from build123d import *

# Parameters (mm, degrees)
F1_DEPTH = 66.675
F2_R     = 1.5875
F2_R_2   = 11.1125
F3_DEPTH = 25.401
F4_R     = 2.8575
F5_DEPTH = 3.556
F6_R     = 3.302
F7_DEPTH = 50.801


with BuildPart() as f1:
    # F0 (on Front) → F1 (new body)
    with BuildSketch(Plane.XZ):
        Polygon((0, 50.8), (0, 0), (25.4, 0), (25.4, 6.35), (6.35, 6.35), (6.35, 50.8), align=None)
    extrude(amount=F1_DEPTH)

    # F2 (on face) → F3 (cut, through all)
    with BuildSketch(Plane(origin=(0, 0, 0), x_dir=(0, -1, 0), z_dir=(-1, 0, 0))):
        with Locations((19.05, 25.4)):
            Circle(F2_R)
        with Locations((33.3375, 39.6875)):
            Circle(F2_R)
        with Locations((33.3375, 25.4)):
            Circle(F2_R_2)
        with Locations((47.625, 25.4)):
            Circle(F2_R)
        with Locations((33.3375, 11.1125)):
            Circle(F2_R)
    extrude(amount=-F3_DEPTH, mode=Mode.SUBTRACT)

    # F4 (on face) → F5 (cut)
    with BuildSketch(Plane(origin=(0, 0, 0), x_dir=(0, -1, 0), z_dir=(-1, 0, 0))):
        with Locations((33.3375, 39.6875)):
            Circle(F4_R)
        with Locations((47.625, 25.4)):
            Circle(F4_R)
        with Locations((33.3375, 11.1125)):
            Circle(F4_R)
        with Locations((19.05, 25.4)):
            Circle(F4_R)
    extrude(amount=-F5_DEPTH, mode=Mode.SUBTRACT)

    # F6 (on face) → F7 (cut, through all)
    with BuildSketch(Plane(origin=(0, 0, 0), x_dir=(1, 0, 0), z_dir=(0, 0, -1))):
        with Locations((12.7, 9.652)):
            Circle(F6_R)
        with Locations((12.7, 57.023)):
            Circle(F6_R)
    extrude(amount=-F7_DEPTH, mode=Mode.SUBTRACT)


solid = f1.part
Verification items for the finished model (mm, model axes). A direction names the side the tool comes from. Give positions to 0.01 mm unless a question says otherwise; leave off trailing zeros. Loops run counter-clockwise (first coordinate to the right, second up) from the corner with the lowest first, then second, coordinate; pieces in that order, holes last.
1. Cross-section at A-A on z = 25.4. Count the separate pieces of the cut face and the enclosed holes in it, and give its area (3 significant figures).
Derived:
separate pieces: 4
enclosed holes: 0
area: 224 mm2
2. Cross-section at C-C on y = -19.05. Record the cut outline in (x, z).
Derived:
outline: (0, 0) - (25.4, 0) - (25.4, 6.35) - (6.35, 6.35) - (6.35, 23.81) - (3.56, 23.81) - (3.56, 22.54) - (0, 22.54) - close; (0, 28.26) - (3.56, 28.26) - (3.56, 26.99) - (6.35, 26.99) - (6.35, 50.8) - (0, 50.8) - close
3. Go/stop test with flat-tipped pins: P1, Ø3.5, axis at y = -47.625, z = 25.4, coming from the -X side; P2, Ø8.5, axis at x = 12.7, y = -57.023, coming from the +Z side; P3, Ø1.9, axis at y = -47.625, z = 25.4, coming from the -X side; P4, Ø5, axis at y = -33.34, z = 11.11, coming from the +X side. Record where each tip stops, or that it passes through.
Derived:
P1: stops at x = 3.56
P2: stops at z = 6.35
P3: passes through
P4: stops at x = 6.35
4. Cross-section at D-D on z = 30.5. Record the cut outline in (x, y) (3 decimals), and give its area (3 significant figures).
Derived:
outline: (0, -66.675) - (6.35, -66.675) - (6.35, -43.211) - (0, -43.211) - close; (0, -23.464) - (6.35, -23.464) - (6.35, 0) - (0, 0) - close
area: 298 mm2
5. Material ranges on probe 1 along X at (y, z) = (-52.5, 13); probe 2 along Y at (x, z) = (5.5, 35) (3 decimals), recorded low to high.
Derived:
probe 1: x = 0 to 6.35
probe 2: y = -66.675 to -38.935, -27.74 to 0
6. Release check for a two-part mould opening along Z. For faces 3 (the flat face through (16, -33, 6.35)), 4 (the cylindrical face through (1.75, -45.36, 23.66)), 5 (the flat face through (0, -25, 37)) record: +Z half, -Z half, draft (parallel to the pull), parting line (faces both ways), or undercut.
Derived:
face 3: +Z half
face 4: undercut
face 5: draft
7. Cross-section at B-B on x = 12.7. Record the cut outline in (y, z) (3 decimals), and give its area (3 significant figures).
Derived:
outline: (-66.675, 0) - (-60.325, 0) - (-60.325, 6.35) - (-66.675, 6.35) - close; (-53.721, 0) - (-12.954, 0) - (-12.954, 6.35) - (-53.721, 6.35) - close; (-6.35, 0) - (0, 0) - (0, 6.35) - (-6.35, 6.35) - close
area: 340 mm2
8. Tool access check on faces 1 (the flat face through (3.556, -20.28, 24.17)), 2 (the cylindrical face through (4.933, -18.843, 26.974)). Record the directions out of +Z, -Z, +X, -X, +Y, -Y that give a thin tool (end or side, any length) a straight path to the whole face; none if there is none.
Derived:
face 1: -X
face 2: +X, -X
